Check sheet for the modelled part. Datum: model origin and axes. Units: mm. A direction names the side the tool comes from. Give positions to 0.01 mm unless a question says otherwise; leave off trailing zeros. Loops run counter-clockwise (first coordinate to the right, second up) from the corner with the lowest first, then second, coordinate; pieces in that order, holes last. Notation, with made-up numbers: (35.25, -21.5) - (46.25, -21.5) arc R31 ccw to (46.25, 13.5) - close; hole circle Ø7 at (86, 55). An arc over 180 degrees is marked (long way). Use CSV: the item, a comma, the result in double quotes.
from build123d import *

# Parameters (mm, degrees)
BOSS_EXTRUDE1_DEPTH   = 0.4
SKETCH1_W             = 76.2
SKETCH1_H             = 234.95
BOSS_EXTRUDE1_2_DEPTH = 0.4
SKETCH2_W             = 1.5875
SKETCH2_H             = 50.8
BOSS_EXTRUDE2_DEPTH   = 0.4


with BuildPart() as part:
    # Sketch1 → Boss-Extrude1 (new body)
    with BuildSketch(Plane.XY):
        Polygon((7.62, 64.577865897), (-14.407538834, 34.29), (7.62, 34.29), align=None)
    extrude(amount=BOSS_EXTRUDE1_DEPTH)



with BuildPart() as body_2:
    # Sketch1 → Boss-Extrude1 2 (new body)
    with BuildSketch(Plane.XY):
        with Locations((0, -31.75)):
            Rectangle(SKETCH1_W, SKETCH1_H)
        Polygon((16.51, 76.2), (16.51, 34.29), (25.4, 34.29), (25.4, 25.4), (16.51, 25.4), (16.51, 12.7), (7.62, 12.7), (7.62, 25.4), (-25.4, 25.4), (-25.4, 34.29), (5.08, 76.2), align=None, mode=Mode.SUBTRACT)
        Polygon((-25.4, 0), (25.4, 0), (-12.506480557, -63.5), (-22.86, -63.5), (9.739573279, -8.89), (-25.4, -8.89), align=None, mode=Mode.SUBTRACT)
        Polygon((-25.4, -76.2), (25.4, -76.2), (-12.506480557, -139.7), (-22.86, -139.7), (9.739573279, -85.09), (-25.4, -85.09), align=None, mode=Mode.SUBTRACT)
    extrude(amount=BOSS_EXTRUDE1_2_DEPTH)


with BuildPart() as part_1:
    add(part.part)

    add(body_2.part)  # Boss-Extrude2 merges body 2
    # Sketch2 → Boss-Extrude2 (add)
    with BuildSketch(Plane.XY.offset(0.4)):
        with Locations((6.82625, 50.8)):
            Rectangle(SKETCH2_W, SKETCH2_H)
    extrude(amount=-BOSS_EXTRUDE2_DEPTH)


solid = part_1.part
1. Scan lines: line 1 along X through (y, z) = (22, 0.15); line 2 along X through (y, z) = (39, 0.1); line 3 along Y through (x, z) = (24, 0.25) (3 decimals). Record each from-to range of solid material in increasing order.
Completed:
line 1,"x = -38.1 to 7.62, 16.51 to 38.1"
line 2,"x = -38.1 to -21.97, -10.98 to 7.62, 16.51 to 38.1"
line 3,"y = -149.225 to -78.545, -76.2 to -2.345, 0 to 25.4, 34.29 to 85.725"
2. Go/stop test with a flat-tipped pin: pin 1 Ø1 at (x, y) = (10, 42) entering from +Z. Record where the tip stops, or that it passes through.
Completed:
pin 1,"passes through"
3. Release check for a two-part mould opening along Y. For faces 3 (the face through (-9, -30, 0.4)), 4 (the face through (6.71, -31.31, 0.2)) record: released by +Y, released by -Y, zero draft, split by the parting line, or undercut.
Completed:
face 3,"zero draft"
face 4,"undercut"
4. Sectioned sample at B-B, the plane x = 12. Record the boundary of the cut face in (y, z) (3 decimals), and give its area (3 significant figures).
Completed:
outline,"(-149.225, 0) - (-98.647, 0) - (-98.647, 0.4) - (-149.225, 0.4) - close; (-76.2, 0) - (-22.447, 0) - (-22.447, 0.4) - (-76.2, 0.4) - close; (0, 0) - (12.7, 0) - (12.7, 0.4) - (0, 0.4) - close; (76.2, 0) - (85.725, 0) - (85.725, 0.4) - (76.2, 0.4) - close"
area,"50.6 mm²"
5. Set-up check for faces 1 (the face through (-9, -30, 0)), 2 (the face through (-6.8, -36.6, 0.2)): record each of +Z, -Z, +X, -X, +Y, -Y from which the full face is reachable in a straight line by a thin tool's end or side.
Completed:
face 1,"-Z, +X, -X, +Y, -Y"
face 2,"+Z, -Z"
6. Sectioned sample at A-A, the plane y = 16.5. Record the boundary of the cut face in (x, z), and give its area (3 significant figures).
Completed:
outline,"(-38.1, 0) - (7.62, 0) - (7.62, 0.4) - (-38.1, 0.4) - close; (16.51, 0) - (38.1, 0) - (38.1, 0.4) - (16.51, 0.4) - close"
area,"26.9 mm²"
7. Sectioned sample at C-C, the plane z = 0.3. State how many separate pieces and enclosed holes the cut face has, and give its area (3 significant figures).
Completed:
separate pieces,"1"
enclosed holes,"4"
area,"14,600 mm²"
8. Sectioned sample at D-D, the plane x = 2. Record the boundary of the cut face in (y, z) (3 decimals), and give its area (3 significant figures).
Completed:
outline,"(-149.225, 0) - (-115.399, 0) - (-115.399, 0.4) - (-149.225, 0.4) - close; (-98.055, 0) - (-85.09, 0) - (-85.09, 0.4) - (-98.055, 0.4) - close; (-76.2, 0) - (-39.199, 0) - (-39.199, 0.4) - (-76.2, 0.4) - close; (-21.855, 0) - (-8.89, 0) - (-8.89, 0.4) - (-21.855, 0.4) - close; (0, 0) - (25.4, 0) - (25.4, 0.4) - (0, 0.4) - close; (34.29, 0) - (56.85, 0) - (56.85, 0.4) - (34.29, 0.4) - close; (71.965, 0) - (85.725, 0) - (85.725, 0.4) - (71.965, 0.4) - close"
area,"63.4 mm²"
